Verification items for the finished model (mm, model axes). A direction names the side the tool comes from. Round coordinates to 2 decimals unless told otherwise and drop trailing zeros. Order: outer loops, then holes, each group sorted by start corner. A loop starts at its lowest first (then second) coordinate and runs counter-clockwise, first axis right, second up. Notation, with made-up numbers: M 48.25,37.5 L 79.25,37.5 A19 cw 79.25,72.5 Z; hole C 45,59.5 d10. An arc over 180 degrees is marked long. Use CSV: the item, a comma, the result in double quotes. Start each with the question number.
Q1. Sectioned sample at D-D (x = -12.5). Enter the section's corners in (y, z), and give its area (3 significant figures).
Q2. Mould release check, pull along X, two halves, no side actions. Record for faces 4 (the face through (0.4, 13, 0)), 5 (the face through (14, 0.4, 0)), 6 (the face through (0, -70.95, -2)), 7 (the face through (-18.59, -47.29, 0.04)): +X half, -X half, draft (parallel to the pull), parting line (faces both ways), or undercut.
Q3. Sectioned sample at A-A (z = -5.5). Enter the section's corners in (x, y).
Q4. Sectioned sample at B-B (y = 19). Enter the section's corners in (x, z).
Q5. Scan lines: line 1 (Y direction, x = 13, z = 1.25); line 2 (Y direction, x = 6, z = -1.25); line 3 (Y direction, x = 5.5, z = -3.5). Record each from-to range of solid material in increasing order.
Q6. Gauge pin test, flat ends, axial feed: pin 1 Ø0.6 at (y, z) = (-69.5, -5) entering from +X; pin 2 Ø3 at (y, z) = (28.5, 1.5) entering from -X; pin 3 Ø2 at (y, z) = (70, -4.5) entering from -X. Record the tip position at first contact, or that the pin passes through.
Q7. Sectioned sample at C-C (x = 15). Enter the section's corners in (y, z).
Q8. Set-up check for faces 1 (the face through (16.07, -16.41, 0.04)), 2 (the face through (0, 68.95, -5)), 3 (the face through (18.907, -46.615, 0.043)): record each of +Z, -Z, +X, -X, +Y, -Y from which the full face is reachable in a straight line by a thin tool's end or side.
Solid Edge part; units mm, degrees
sketch "Sketch1" plane through (0, 0, 0) normal (0, 0, -1) x (-1, 0, 0)
  line L0 (30, -22.9524) -> (30, 22.9378)
  line L1 (30, 22.9378) -> (7.5, 70.95)
  line L2 (7.5, 70.95) -> (-7.5, 70.95)
  line L3 (-7.5, 70.95) -> (-30, 22.9378)
  line L4 (-30, 22.9378) -> (-30, -22.9524)
  line L5 (-30, -22.9524) -> (-7.5, -70.95)
  line L6 (-7.5, -70.95) -> (7.5, -70.95)
  line L7 (7.5, -70.95) -> (30, -22.9524)
  line L8 (-0.4, 4.2876) -> (-0.4, 22.9378)
  arc A0 (-3.9818, 0.4) -> (-0.4, 4.2876) centre (0.3962, -0.0398) cw
  line L9 (-22.9964, 0.4) -> (-3.9818, 0.4)
  arc A1 (-0.4, 22.9378) -> (-22.9964, 0.4) centre (-0.0011, -0.0586) ccw
  line L10 (-22.9964, -0.4) -> (-3.9818, -0.4)
  arc A2 (-0.4, -22.9524) -> (-22.9964, -0.4) centre (-0.0008, 0.044) cw
  line L11 (-0.4, -4.3267) -> (-0.4, -22.9524)
  arc A3 (-3.9818, -0.4) -> (-0.4, -4.3267) centre (0.4, 0) ccw
  arc A4 (0.4, 22.9378) -> (0.4, -22.9524) centre (-1.1861, -0.0073) cw
  line L12 (0.4, 3.6) -> (0.4, 22.9378)
  arc A5 (0.4, -3.6) -> (0.4, 3.6) centre (0.4, 0) cw
  line L13 (0.4, -22.9524) -> (0.4, -3.6)
extrude "ExtrudedProtrusion_3" add sketch "Sketch1" along normal mid plane 6.2
sketch "Sketch2" plane through (0, 0, -3.1) normal (0, 0, -1) x (0, 1, 0)
  line L0 (-68.95, -7.5) -> (-70.95, -7.5)
  line L1 (-70.95, -7.5) -> (-70.95, 7.5)
  line L2 (-70.95, 7.5) -> (-68.95, 7.5)
  line L3 (-68.95, 7.5) -> (-68.95, -7.5)
  line L4 (68.95, 7.5) -> (68.95, -7.5)
  line L5 (68.95, -7.5) -> (70.95, -7.5)
  line L6 (70.95, -7.5) -> (70.95, 7.5)
  line L7 (70.95, 7.5) -> (68.95, 7.5)
extrude "ExtrudedProtrusion_4" add sketch "Sketch2" along normal blind 3.9
properties material "PLA Filament"
Verdict:
1,outline,"M -60.28,-3.1 L -18.49,-3.1 L -18.49,3.1 L -60.28,3.1 Z; M 18.48,-3.1 L 60.28,-3.1 L 60.28,3.1 L 18.48,3.1 Z"
1,area,"518 mm²"
2,face 4,"undercut"
2,face 5,"undercut"
2,face 6,"draft"
2,face 7,"-X half"
3,outline,"M -7.5,-70.95 L 7.5,-70.95 L 7.5,-68.95 L -7.5,-68.95 Z; M -7.5,68.95 L 7.5,68.95 L 7.5,70.95 L -7.5,70.95 Z"
4,outline,"M -30,-3.1 L -11.76,-3.1 L -11.76,3.1 L -30,3.1 Z; M -0.4,-3.1 L 0.4,-3.1 L 0.4,3.1 L -0.4,3.1 Z; M 12.88,-3.1 L 30,-3.1 L 30,3.1 L 12.88,3.1 Z"
5,line 1,"y = -59.22 to -18.93, -0.4 to 0.4, 18.92 to 59.21"
5,line 2,"y = -70.95 to -22.16, -0.4 to 0.4, 22.15 to 70.95"
5,line 3,"y = -70.95 to -68.95, 68.95 to 70.95"
6,pin 1,"stops at x = 7.5"
6,pin 2,"stops at x = -28.1"
6,pin 3,"stops at x = -7.5"
7,outline,"M -54.95,-3.1 L -17.39,-3.1 L -17.39,3.1 L -54.95,3.1 Z; M -0.4,-3.1 L 0.4,-3.1 L 0.4,3.1 L -0.4,3.1 Z; M 17.38,-3.1 L 54.95,-3.1 L 54.95,3.1 L 17.38,3.1 Z"
8,face 1,"+Z, -Z"
8,face 2,"-Z, +X, -X"
8,face 3,"+Z, -Z, +X, -Y"
